Design review of the part built by this model. Coordinates are the model's own, in mm. A direction names the side the tool comes from. Give positions to 0.01 mm unless a question says otherwise; leave off trailing zeros. Write each loop counter-clockwise with the first axis right and the second up, starting at its lowest first coordinate (ties: lowest second). Pieces come first, ordered by that corner, then holes. Notation, with made-up numbers: (9, 15) -> (64, 15) arc R20 cw to (64, 24) -> close; hole circle Ø1 at (32.5, 89). An arc over 180 degrees is marked (long way). Put each result on its own line as item: value. Start each with the question number.
from build123d import *

# Parameters (mm, degrees)
BOSS_EXTRUDE1_DEPTH = 12.7
SKETCH2_W           = 12.7
SKETCH2_H           = 19.05
CUT_EXTRUDE1_DEPTH  = 13.7


with BuildPart() as part:
    # Sketch1 → Boss-Extrude1 (new body)
    with BuildSketch(Plane.XY):
        Polygon((0, -215.9), (8.89, -215.9), (72.148675035, -152.641324965), (83.080541238, -152.641324965), (83.080541238, 0), (76.730541238, 0), (0, 0), align=None)
    extrude(amount=BOSS_EXTRUDE1_DEPTH)

    # Sketch2 → Cut-Extrude1 (cut, through all)
    with BuildSketch(Plane.XY.offset(12.7)):
        with Locations((6.35, -9.525)):
            Rectangle(SKETCH2_W, SKETCH2_H)
        with Locations((6.35, -206.375)):
            Rectangle(SKETCH2_W, SKETCH2_H)
    extrude(amount=-CUT_EXTRUDE1_DEPTH, mode=Mode.SUBTRACT)


solid = part.part
Q1. Take a section at A-A on z = 4. Give the boundary of the cut face in (x, y).
Q2. For pin 1 (6.5 mm diameter, centred on y = -202, z = 6.5, fed in from -X); pin 2 (6.5 mm diameter, centred on x = 6.5, z = 3, fed in from -Y); pin 3 (2 mm diameter, centred on x = 30.5, z = 1.5, fed in from -Y), all flat-tipped, find the tip position at first contact; note any pin that passes through.
Q3. Take a section at C-C on x = 77. Give the boundary of the cut face in (y, z).
Q4. Machinability: for faces 1 (the face through (78, -152.641, 6)), 2 (the face through (12.7, -10, 6)), 3 (the face through (6, -196.85, 6)), which of the approach directions +Z, -Z, +X, -X, +Y, -Y give a long, thin tool a straight path to every point of the face, cutting with its end or side? Answer none if there is none.
Q5. To check wall thickness, follow probe 1 along Y at (x, z) = (73.5, 1); probe 2 along Y at (x, z) = (65.5, 4); probe 3 along X at (y, z) = (-202, 4.75). State the ranges of each line that lie inside material, in increasing order. Write a range as from..to.
Q6. Take a section at B-B on x = 54.5. Give the boundary of the cut face in (y, z), then the cut area to 3 significant figures.
Result:
1. outline: (0, -196.85) -> (12.7, -196.85) -> (12.7, -212.09) -> (72.15, -152.64) -> (83.08, -152.64) -> (83.08, 0) -> (12.7, 0) -> (12.7, -19.05) -> (0, -19.05) -> close
2. pin 1: stops at x = 12.7
2. pin 2: stops at y = -196.85
2. pin 3: stops at y = -195.29
3. outline: (-152.64, 0) -> (0, 0) -> (0, 12.7) -> (-152.64, 12.7) -> close
4. face 1: +Z, -Z, +X, -Y
4. face 2: +Z, -Z, -X, +Y
4. face 3: +Z, -Z, -X, -Y
5. probe 1: y = -152.64..0
5. probe 2: y = -159.29..0
5. probe 3: x = 12.7..22.79
6. outline: (-170.29, 0) -> (0, 0) -> (0, 12.7) -> (-170.29, 12.7) -> close
6. area: 2,160 mm^2
